Verification items for this drawing (mm, ordinates from the low corner). A direction names the side the tool comes from. Give positions to 0.01 mm unless a question says otherwise; leave off trailing zeros. Write each loop counter-clockwise with the first axis right and the second up, starting at its lowest first coordinate (ties: lowest second). Pieces come first, ordered by that corner, then holes. Notation, with made-up numbers: M 12.25,-15.75 L 27.25,-15.75 A34 cw 27.25,19.25 Z; hole C 11.5,24.5 d8. An arc over 180 degrees is marked long. Use one line per item in the form item = value. Start each with the question number.
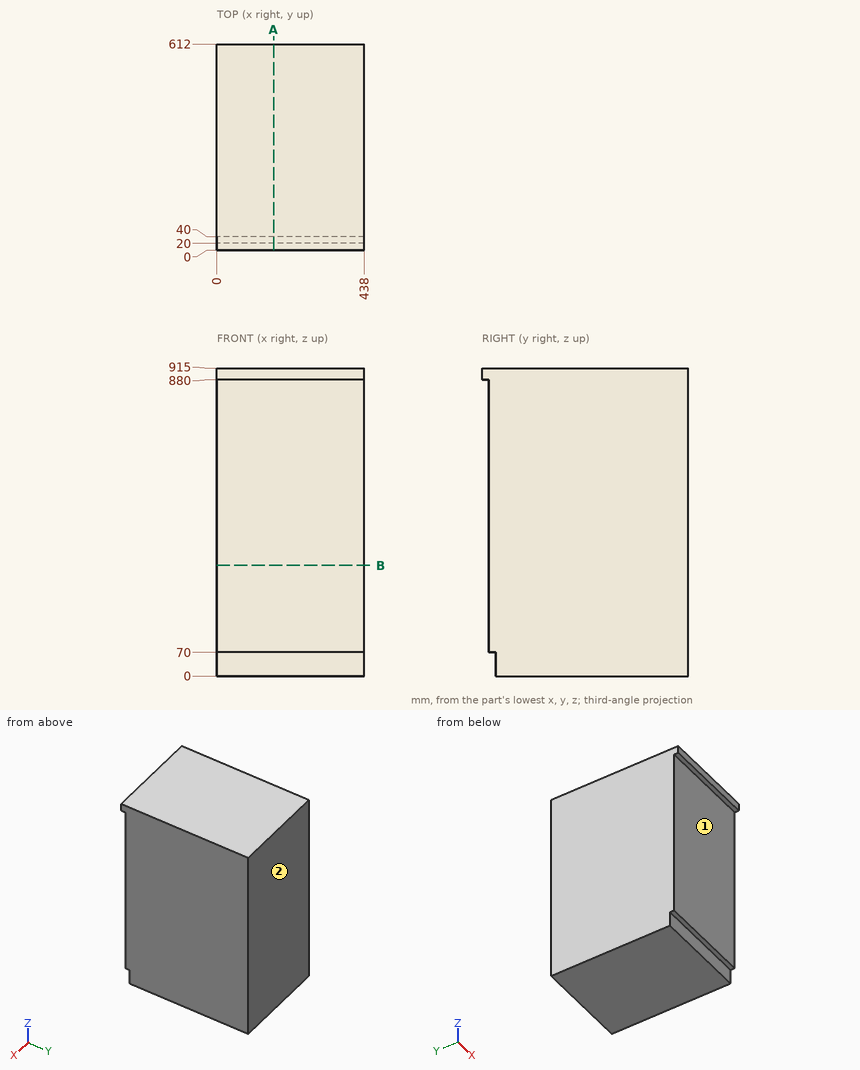
(1) Sectioned sample at A-A, the plane x = 169. Record the boundary of the cut face in (y, z).
(2) Tool access check on the marked faces 1 and 2. Record the directions out of +Z, -Z, +X, -X, +Y, -Y that give a thin tool (end or side, any length) a straight path to the whole face; none if there is none.
(3) Sectioned sample at B-B, the plane z = 328.5. Record the boundary of the cut face in (x, y).
(4) Depth check by flat-ended pin: pin 1 (3 mm diameter, centred on x = 267.5, z = 684, fed in from -Y); pin 2 (22 mm diameter, centred on x = 256.5, y = 10.5, fed in from -Z). Enter the tip coordinate at first touch or a pass-through.
(5) Thickness scan on probe 1 along Y at (x, z) = (160.5, 823); probe 2 along Y at (x, z) = (178.5, 44.5). Record the ranges inside material, lowest first. Write a range as [from, to].
Numbers:
q1.outline = M 0,880 L 20,880 L 20,70 L 40,70 L 40,0 L 612,0 L 612,915 L 0,915 Z
q2.face_1 = -Z, +X, -X, -Y
q2.face_2 = +Z, -Z, +X, -X, +Y
q3.outline = M 0,20 L 438,20 L 438,612 L 0,612 Z
q4.pin_1 = 20
q4.pin_2 = 70
q5.probe_1 = [20, 612]
q5.probe_2 = [40, 612]
